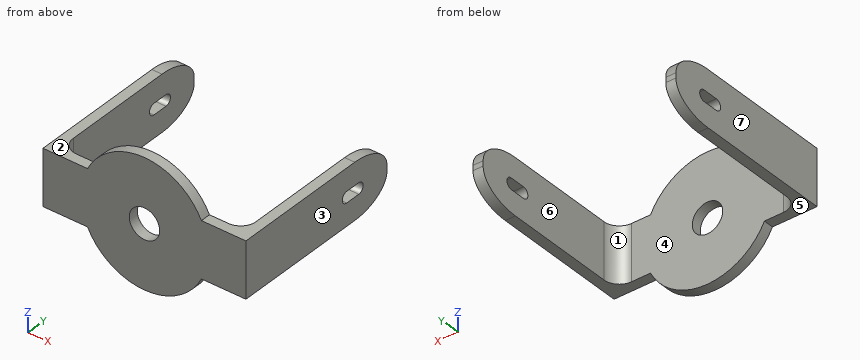
from build123d import *

# Parameters (mm, degrees)
SKETCH_1_R               = 3
EXTRUDE_1_DEPTH          = 2
SKETCH_2_W               = 2
SKETCH_2_H               = 11
EXTRUDE_2_DEPTH          = 35
FILLET_1_SIZE            = 8
FILLET_1_SIZE_2          = 5
CUT_EXTRUDE_1_DEPTH      = 55.600824307
CUT_EXTRUDE_1_DEPTH_BACK = 55.600824307
FILLET_2_R               = 3


with BuildPart() as part:
    # 草图1 → 凸台-拉伸1 (new body)
    with BuildSketch(Plane(origin=(0, 0, 0), x_dir=(1, 0, 0), z_dir=(0, 1, 0))):
        with BuildLine():
            Line((-11.22497216, 5.5), (-18, 5.5))
            Line((-18, 5.5), (-18, -5.5))
            Line((-18, -5.5), (-11.22497216, -5.5))
            ThreePointArc((-11.22497216, -5.5), (0, -12.5), (11.22497216, -5.5))
            Line((11.22497216, -5.5), (18, -5.5))
            Line((18, -5.5), (18, 5.5))
            Line((18, 5.5), (11.22497216, 5.5))
            ThreePointArc((11.22497216, 5.5), (0, 12.5), (-11.22497216, 5.5))
        make_face()
        with Locations(Location((0, 0, 0), (0, 0, 270))):
            Circle(SKETCH_1_R, mode=Mode.SUBTRACT)
    extrude(amount=EXTRUDE_1_DEPTH)

    # 草图2 → 凸台-拉伸2 (add)
    with BuildSketch(Plane(origin=(0, 0, 0), x_dir=(1, 0, 0), z_dir=(0, 1, 0))):
        with Locations((-19, 0)):
            Rectangle(SKETCH_2_W, SKETCH_2_H)
        with Locations((19, 0)):
            Rectangle(SKETCH_2_W, SKETCH_2_H)
    extrude(amount=EXTRUDE_2_DEPTH)

    # 圆角1
    # an asymmetric fillet: 8, 5 mm, written as the material it takes off along each edge
    with BuildSketch(Plane(origin=(40, 35, -5.5), x_dir=(0, -1, 0), z_dir=(-1, 0, 0)), Plane(origin=(2, 35, -5.5), x_dir=(0, -1, 0), z_dir=(-1, 0, 0)), Plane(origin=(-40, 35, 5.5), x_dir=(0, -1, 0), z_dir=(1, 0, 0))) as fillet_1_piece_1:
        with BuildLine():
            Bezier((FILLET_1_SIZE, 0), (0, 0), (0, FILLET_1_SIZE_2), weights=[1, 0.707106781, 1])
            Line((0, FILLET_1_SIZE_2), (0, 0))
            Line((0, 0), (FILLET_1_SIZE, 0))
        make_face()
    extrude(amount=42, mode=Mode.SUBTRACT)
    with BuildSketch(Plane(origin=(-2, 35, 5.5), x_dir=(0, 0, -1), z_dir=(1, 0, 0))) as fillet_1_piece_2:
        with BuildLine():
            Bezier((FILLET_1_SIZE_2, 0), (0, 0), (0, -FILLET_1_SIZE), weights=[1, 0.707106781, 1])
            Line((0, -FILLET_1_SIZE), (0, 0))
            Line((0, 0), (FILLET_1_SIZE_2, 0))
        make_face()
    extrude(amount=42, mode=Mode.SUBTRACT)

    # 草图3 → 切除-拉伸1 (cut, two sides: drawn at the far end of the back side and taken through both)
    with BuildSketch(Plane.ZY.offset(20).offset(-CUT_EXTRUDE_1_DEPTH_BACK)):
        with BuildLine():
            Line((1.1, 28), (1.1, 25))
            ThreePointArc((1.1, 25), (0, 23.9), (-1.1, 25))
            Line((-1.1, 25), (-1.1, 28))
            ThreePointArc((-1.1, 28), (0, 29.1), (1.1, 28))
        make_face()
    extrude(amount=CUT_EXTRUDE_1_DEPTH + CUT_EXTRUDE_1_DEPTH_BACK, mode=Mode.SUBTRACT)

    # 圆角2
    fillet_2_edges = [part.edges().sort_by_distance(p)[0] for p in [
        (18, 2, 0),
        (-18, 2, 0),
    ]]
    fillet(fillet_2_edges, radius=FILLET_2_R)


solid = part.part
Part model, mm, in its own coordinate system. Face numbers are marked on the shaded views. A direction names the side the tool comes from. Give positions to 0.01 mm unless a question says otherwise; leave off trailing zeros. Order: outer loops, then holes, each group sorted by start corner. A loop starts at its lowest first (then second) coordinate and runs counter-clockwise, first axis right, second up. Notation, with made-up numbers: (-37.75, 28) -> (-25.75, 28) arc R27 ccw to (-25.75, 61) -> close; hole circle Ø3 at (-6, 26). An arc over 180 degrees is marked (long way). Use one line per item in the form item = value.
(1) Pull direction X, two halves, no side cores. Call the marked faces 4, 5, 6 and 7: +X half, -X half, draft (parallel to the pull), parting line (faces both ways), or undercut.
Solution:
face_4 = undercut
face_5 = draft
face_6 = undercut
face_7 = -X half
(2) Drill centre lines: line 1 (X direction, y = 0.8, z = 0); line 2 (X direction, y = 13, z = -4.25); line 3 (Y direction, x = -1.5, z = -9.75). Where is each one in solid material? Low to high. Write a range as from..to.
Solution:
line_1 = -20..-3, 3..20
line_2 = -20..-18, 18..20
line_3 = 0..2
(3) Saw through at A-A (y = 12.5). Write the cut outline in (x, z), then the cut area to 3 significant figures.
Solution:
outline = (-20, -5.5) -> (-18, -5.5) -> (-18, 5.5) -> (-20, 5.5) -> close; (18, -5.5) -> (20, -5.5) -> (20, 5.5) -> (18, 5.5) -> close
area = 44.0 mm²
(4) Saw through at C-C (x = 1). Write the cut outline in (y, z).
Solution:
outline = (0, -12.46) -> (2, -12.46) -> (2, -2.83) -> (0, -2.83) -> close; (0, 2.83) -> (2, 2.83) -> (2, 12.46) -> (0, 12.46) -> close
(5) Flat gauge pins, fed straight in: P1, Ø5, axis at x = -15, y = 7, coming from the +Z side; P2, Ø2, axis at x = 19.5, y = 26.5, coming from the +Z side; P3, Ø1, axis at x = 19, y = 26, coming from the -Z side; P4, Ø8, axis at x = 0, z = 0, coming from the +Y side. Where does each tip first touch, or does it go through?
Solution:
P1 = through
P2 = 5.5
P3 = -5.5
P4 = 2
(6) Tool access for the marked faces 1, 2 and 3: list every direction of +Z, -Z, +X, -X, +Y, -Y with a clear straight run to the whole face (end or side of a thin tool).
Solution:
face_1 = +Z, -Z, +Y
face_2 = +Z, -X, +Y, -Y
face_3 = +Z, -Z, +X, +Y, -Y
(7) Saw through at D-D (x = -13). Write the cut outline in (y, z), then the cut area to 3 significant figures.
Solution:
outline = (0, -5.5) -> (2, -5.5) -> (2, 5.5) -> (0, 5.5) -> close
area = 22.0 mm²
(8) Saw through at B-B (z = 0). Write the cut outline in (x, y).
Solution:
outline = (-20, 0) -> (-3, 0) -> (-3, 2) -> (-15, 2) arc R3 cw to (-18, 5) -> (-18, 23.9) -> (-20, 23.9) -> close; (-20, 29.1) -> (-18, 29.1) -> (-18, 35) -> (-20, 35) -> close; (3, 0) -> (20, 0) -> (20, 23.9) -> (18, 23.9) -> (18, 5) arc R3 cw to (15, 2) -> (3, 2) -> close; (18, 29.1) -> (20, 29.1) -> (20, 35) -> (18, 35) -> close
